Answer from the drawing. Dimensions are ordinates in mm from the lowest x, y and z of the part. A direction names the side the tool comes from. Round coordinates to 2 decimals unless told otherwise and drop trailing zeros. Write each loop counter-clockwise with the first axis right and the second up, starting at its lowest first coordinate (ties: lowest second). Pieces come first, ordered by that corner, then holes.
1. Flat-ended cylindrical pins translate along their axes: pin 1 Ø5 at (x, y) = (116.5, 3) entering from +Z; pin 2 Ø12 at (x, z) = (143.5, 86.5) entering from -Y. Find the tip coordinate at first contact, or state that the pin passes through.
2. Determine the mould class of the marked faces 1, 2, 3 and 4 for opening direction Y: pulls with the +Y half, pulls with the -Y half, needs draft (parallel to the pull), parting line crosses it, or undercut.
3. Straight lines are drawn through the part: probe 1 along Y at (x, z) = (88.5, 4); probe 2 along X at (y, z) = (18, 79) (1 decimal). For each, find the intervals that lie inside material, in ascending order.
4. Find section A-A (x = 85). Write down the section's boundary in (y, z), and give its area (3 significant figures).
5. Find section D-D (y = 45.5). Write down the section's boundary in (x, z) (1 decimal).
6. A tool of negligible diameter and unlimited length cuts with its end or side. For the marked faces 5 and 6, from which of +Z, -Z, +X, -X, +Y, -Y can it reach the whole face along a straight path? Write none if from no direction.
7. Find section B-B (z = 11). Write down the section's boundary in (x, y) (1 decimal).
8. Find section C-C (y = 81). Write down the section's boundary in (x, z) (1 decimal), and give its area (3 significant figures).
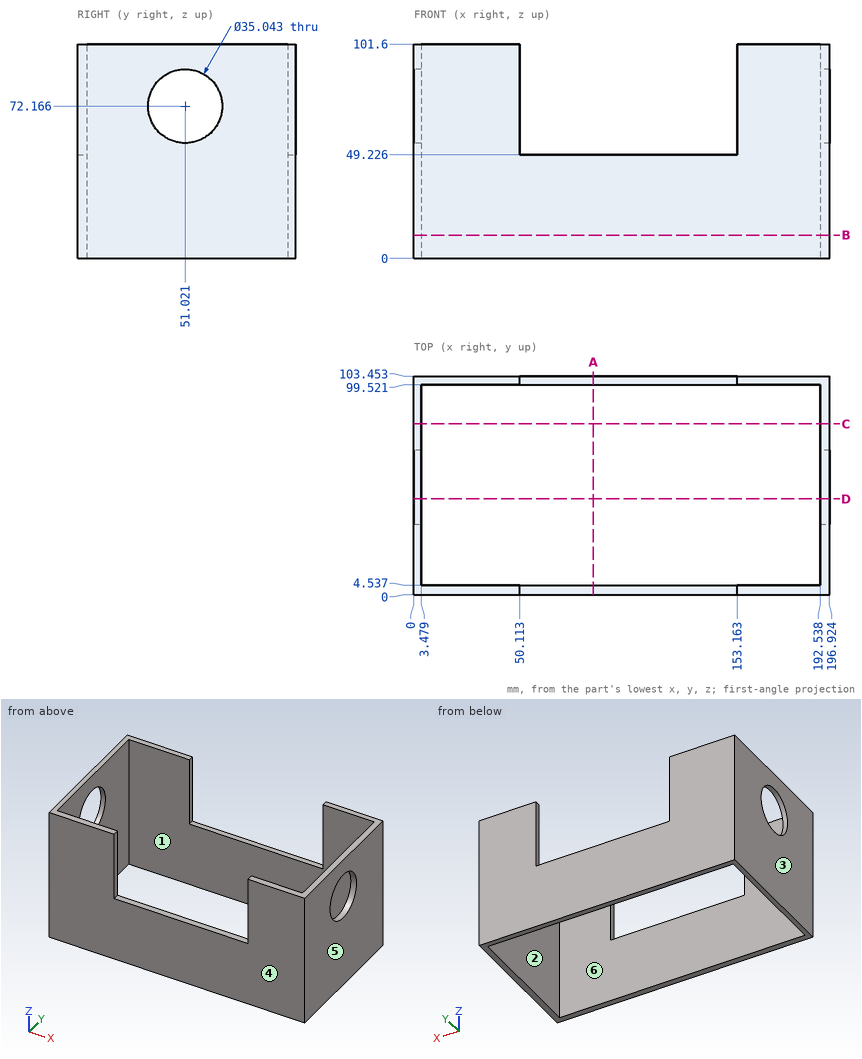
Worked answers:
1. pin 1: stops at z = 49.23
1. pin 2: passes through
2. face 1: undercut
2. face 2: undercut
2. face 3: needs draft
2. face 4: pulls with the -Y half
3. probe 1: y = 0 to 4.54, 99.52 to 103.45
3. probe 2: x = 0 to 3.5, 192.5 to 196.9
4. outline: (0, 0) - (4.54, 0) - (4.54, 49.23) - (0, 49.23) - close; (99.52, 0) - (103.45, 0) - (103.45, 49.23) - (99.52, 49.23) - close
4. area: 417 mm2
5. outline: (0, 0) - (3.5, 0) - (3.5, 55.5) - (0, 55.5) - close; (0, 88.8) - (3.5, 88.8) - (3.5, 101.6) - (0, 101.6) - close; (192.5, 0) - (196.9, 0) - (196.9, 55.5) - (192.5, 55.5) - close; (192.5, 88.8) - (196.9, 88.8) - (196.9, 101.6) - (192.5, 101.6) - close
6. face 5: +Z, -Z, +X, +Y, -Y
6. face 6: +Z, -Z
7. outline: (0, 0) - (196.9, 0) - (196.9, 103.5) - (0, 103.5) - close; hole (3.5, 4.5) - (192.5, 4.5) - (192.5, 99.5) - (3.5, 99.5) - close
8. outline: (0, 0) - (3.5, 0) - (3.5, 101.6) - (0, 101.6) - close; (192.5, 0) - (196.9, 0) - (196.9, 101.6) - (192.5, 101.6) - close
8. area: 799 mm2
